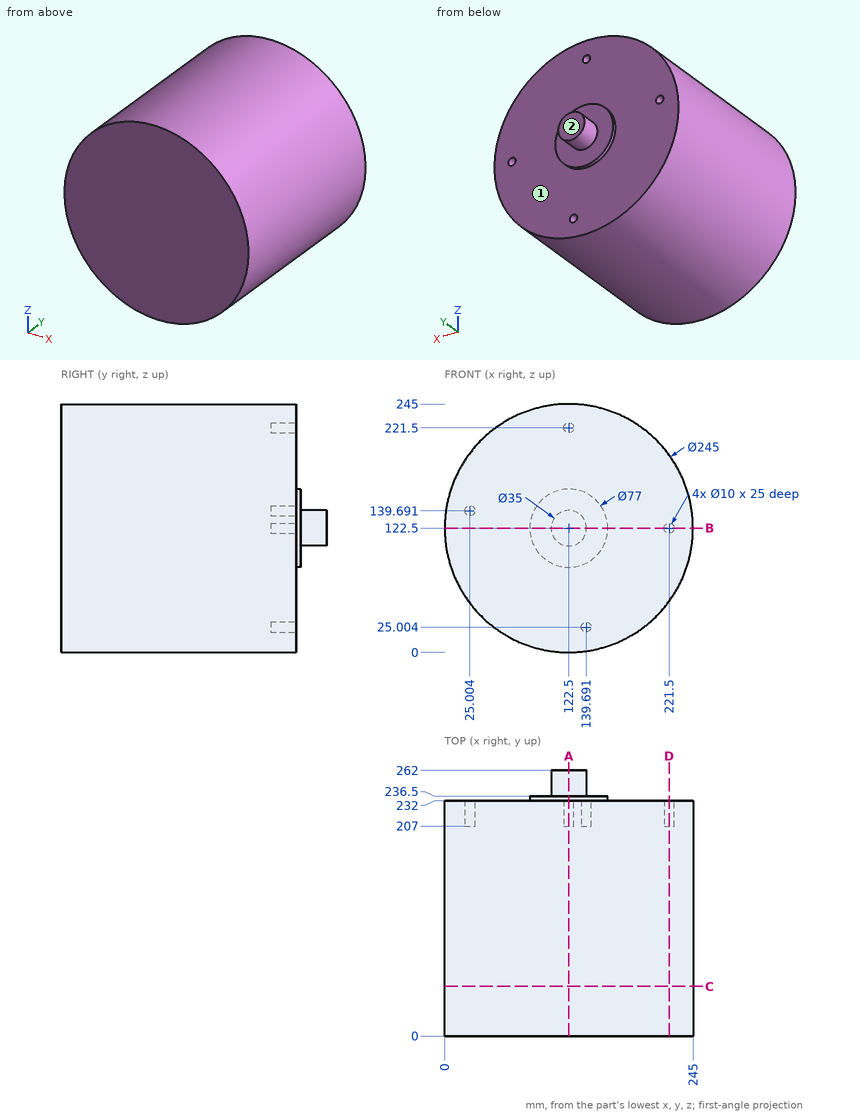
Geometry check sheet. Reference: drawing and pictorial views, mm from the part's lowest x, y, z. A direction names the side the tool comes from. Coordinates: 2 decimals unless noted, no trailing zeros. Loops run counter-clockwise (first coordinate to the right, second up) from the corner with the lowest first, then second, coordinate; pieces in that order, holes last. Notation, with made-up numbers: (1.25, -15.75) - (28.25, -15.75) arc R23 ccw to (28.25, -2.75) - close; hole circle Ø3 at (-25, 36). An arc over 180 degrees is marked (long way). Return JSON: item names as keys, results as strings.
1. Go/stop test with flat-tipped pins: pin 1 (1 mm diameter, centred on y = 83.5, z = 95.5, fed in from +X); pin 2 (11 mm diameter, centred on x = 223, z = 122.5, fed in from +Y); pin 3 (9 mm diameter, centred on x = 122.5, z = 221.5, fed in from +Y); pin 4 (16 mm diameter, centred on x = 221.5, z = 122.5, fed in from -Y). Record where each tip stops, or that it passes through.
Established:
{"pin 1": "stops at x = 242.1", "pin 2": "stops at y = 232", "pin 3": "stops at y = 207", "pin 4": "stops at y = 0"}
2. Thickness scan on L1, parallel to Y at x = 235.5, z = 149.5; L2, parallel to Y at x = 96.5, z = 135; L3, parallel to Z at x = 221, y = 216 (1 decimal). Record the ranges inside material, lowest first.
Established:
{"L1": "y = 0 to 232", "L2": "y = 0 to 236.5", "L3": "z = 49.7 to 117.5, 127.5 to 195.3"}
3. Section check A-A, the plane x = 122.5. Record the boundary of the cut face in (y, z).
Established:
{"outline": "(0, 0) - (232, 0) - (232, 84) - (236.5, 84) - (236.5, 105) - (262, 105) - (262, 140) - (236.5, 140) - (236.5, 161) - (232, 161) - (232, 216.5) - (207, 216.5) - (207, 226.5) - (232, 226.5) - (232, 245) - (0, 245) - close"}
4. Section check D-D, the plane x = 221.5. Record the boundary of the cut face in (y, z), then the cut area to 3 significant figures.
Established:
{"outline": "(0, 50.35) - (232, 50.35) - (232, 117.5) - (207, 117.5) - (207, 127.5) - (232, 127.5) - (232, 194.65) - (0, 194.65) - close", "area": "33,200 mm2"}
5. Section check B-B, the plane z = 122.5. Record the boundary of the cut face in (x, y).
Established:
{"outline": "(0, 0) - (245, 0) - (245, 232) - (226.5, 232) - (226.5, 207) - (216.5, 207) - (216.5, 232) - (161, 232) - (161, 236.5) - (140, 236.5) - (140, 262) - (105, 262) - (105, 236.5) - (84, 236.5) - (84, 232) - (0, 232) - close"}
6. Section check C-C, the plane y = 49. Record the boundary of the cut face in (x, z), then the cut area to 3 significant figures.
Established:
{"outline": "circle Ø245 at (122.5, 122.5)", "area": "47,100 mm2"}
7. Tool access check on the marked faces 1 and 2. Record the directions out of +Z, -Z, +X, -X, +Y, -Y that give a thin tool (end or side, any length) a straight path to the whole face; none if there is none.
Established:
{"face 1": "+Y", "face 2": "+Z, -Z, +X, -X, +Y"}
